The model under review builds one solid part; all positions refer to its coordinate system, in mm. Give positions to 0.01 mm unless a question says otherwise; leave off trailing zeros.
Autodesk Inventor part; units mm, degrees
ref_plane "YZ Plane" through (0, 0, 0) normal (1, 0, 0) x (0, 1, 0)
ref_plane "XZ Plane" through (0, 0, 0) normal (0, 1, 0) x (-1, 0, 0)
ref_plane "XY Plane" through (0, 0, 0) normal (0, 0, 1) x (1, 0, 0)
sketch "Sketch1" plane through (0, 0, 0) normal (0, 0, 1) x (1, 0, 0)
  line L0 (-412.8165, 301.8597) -> (87.1835, 301.8597)
  line L1 (-427.8165, 301.8597) -> (-412.8165, 301.8597)
  line L2 (-427.8165, 286.8597) -> (-427.8165, 301.8597)
  line L3 (-427.8165, -73.1403) -> (-427.8165, 286.8597)
  line L4 (-412.8165, 286.8597) -> (-427.8165, 286.8597)
  line L5 (-412.8165, 286.8597) -> (-427.8165, 286.8597)
  line L6 (-412.8165, 301.8597) -> (-412.8165, 286.8597)
  line L7 (-427.8165, 301.8597) -> (-412.8165, 301.8597)
  line L8 (-427.8165, 286.8597) -> (-427.8165, 301.8597)
  line L9 (-412.8165, -88.1403) -> (-412.8165, -73.1403)
  line L10 (-412.8165, -73.1403) -> (-427.8165, -73.1403)
  line L11 (-427.8165, -88.1403) -> (-427.8165, -73.1403)
  line L12 (-412.8165, -88.1403) -> (-427.8165, -88.1403)
  line L13 (-412.8165, -73.1403) -> (-412.8165, 286.8597)
  line L14 (87.1835, -73.1403) -> (-412.8165, -73.1403)
  line L15 (87.1835, -88.1403) -> (-412.8165, -88.1403)
  line L16 (102.1835, -88.1403) -> (102.1835, -73.1403)
  line L17 (102.1835, -73.1403) -> (87.1835, -73.1403)
  line L18 (87.1835, -88.1403) -> (87.1835, -73.1403)
  line L19 (102.1835, -88.1403) -> (87.1835, -88.1403)
  line L20 (87.1835, -73.1403) -> (87.1835, 286.8597)
  line L21 (102.1835, -73.1403) -> (102.1835, 286.8597)
  line L22 (87.1835, 286.8597) -> (102.1835, 286.8597)
  line L23 (102.1835, 286.8597) -> (102.1835, 301.8597)
  line L24 (87.1835, 301.8597) -> (102.1835, 301.8597)
  line L25 (87.1835, 286.8597) -> (87.1835, 301.8597)
  line L26 (87.1835, 286.8597) -> (-412.8165, 286.8597)
  line L27 (-312.8165, -73.1403) -> (-312.8165, 286.8597)
  line L28 (-297.8165, -73.1403) -> (-297.8165, 286.8597)
  line L29 (-12.8165, -73.1403) -> (-12.8165, 286.8597)
  line L30 (-27.8165, -73.1403) -> (-27.8165, 286.8597)
  line L31 (-425.8165, -71.1403) -> (-410.8165, -71.1403)
  line L32 (-410.8165, -71.1403) -> (-410.8165, -86.1403)
  line L33 (-410.8165, -86.1403) -> (85.1835, -86.1403)
  line L34 (85.1835, -86.1403) -> (85.1835, -71.1403)
  line L35 (85.1835, -71.1403) -> (100.1835, -71.1403)
  line L36 (100.1835, -71.1403) -> (100.1835, 284.8597)
  line L37 (100.1835, 284.8597) -> (85.1835, 284.8597)
  line L38 (85.1835, 284.8597) -> (85.1835, 299.8597)
  line L39 (85.1835, 299.8597) -> (-410.8165, 299.8597)
  line L40 (-410.8165, 299.8597) -> (-410.8165, 284.8597)
  line L41 (-410.8165, 284.8597) -> (-425.8165, 284.8597)
  line L42 (-425.8165, 284.8597) -> (-425.8165, -71.1403)
  point P0 (0, 0)
  dimension "d2" = 2
  dimension "d3" = 2
  dimension "d4" = 2
  dimension "d5" = 2
  dimension "d6" = 2
  dimension "d7" = 2
  dimension "d8" = 2
  dimension "d9" = 2
  dimension "d10" = 2
  dimension "d11" = 2
  dimension "d12" = 2
  dimension "d13" = 2
extrude "Extrusion1" add sketch "Sketch1" along normal blind 3 contours L41 L40 L26 L27 L14 L32 L31 L13 | L13 L31 L42 L41 | L40 L39 L38 L26 | L37 L36 L35 L20 | L20 L35 L34 L14 L29 L26 L38 L37 | L26 L28 L14 L27 | L29 L14 L30 L26 | L26 L30 L14 L28 | L14 L34 L33 L32
sketch "Sketch3" plane through (0, 0, 3) normal (0, 0, 1) x (1, 0, 0)
  line L0 (100.1835, -71.1403) -> (100.1835, 284.8597)
  line L1 (-425.8165, 284.8597) -> (-425.8165, -71.1403)
  line L2 (-425.8165, -71.1403) -> (-410.8165, -71.1403)
  line L3 (-410.8165, 284.8597) -> (-425.8165, 284.8597)
  line L4 (85.1835, -86.1403) -> (85.1835, -71.1403)
  line L5 (-410.8165, 299.8597) -> (-410.8165, 284.8597)
  line L6 (-410.8165, -86.1403) -> (85.1835, -86.1403)
  line L7 (85.1835, 299.8597) -> (-410.8165, 299.8597)
  point P0 (0, 0)
  point P1 (94.6835, -21.1403)
  point P2 (94.6835, 106.8597)
  point P3 (94.6835, 234.8597)
  point P4 (-420.3165, 234.8597)
  point P5 (-420.3165, 106.8597)
  point P6 (-420.3165, -21.1403)
  point P7 (35.1835, -80.6403)
  point P8 (-94.8165, -80.6403)
  point P9 (-230.8165, -80.6403)
  point P10 (-360.8165, -80.6403)
  point P11 (-360.8165, 294.3597)
  point P12 (-230.8165, 294.3597)
  point P13 (-94.8165, 294.3597)
  point P14 (35.1835, 294.3597)
  dimension "d18" = 5.5
  dimension "d19" = 5.5
  dimension "d20" = 50
  dimension "d21" = 50
  dimension "d22" = 356
  dimension "d23" = 178
  dimension "d24" = 50
  dimension "d25" = 50
  dimension "d26" = 5.5
  dimension "d27" = 5.5
  dimension "d28" = 180
  dimension "d29" = 180
hole "FrameMountHoles" at (94.6835, -21.1403, 3) at (94.6835, 106.8597, 3) at (94.6835, 234.8597, 3) at (-420.3165, 234.8597, 3) at (-420.3165, 106.8597, 3) at (-420.3165, -21.1403, 3) at (35.1835, -80.6403, 3) at (-94.8165, -80.6403, 3) at (-230.8165, -80.6403, 3) at (-360.8165, -80.6403, 3) at (-360.8165, 294.3597, 3) at (-230.8165, 294.3597, 3) at (-94.8165, 294.3597, 3) at (35.1835, 294.3597, 3) direction (0, 0, -1) diameter 4 depth 8 tip angle 118
sketch "Sketch10" plane through (0, 0, 3) normal (0, 0, 1) x (1, 0, 0)
  circle A0 centre (-94.8165, 294.3597) radius 2
  circle A1 centre (-360.8165, 294.3597) radius 2
  circle A2 centre (-230.8165, -80.6403) radius 2
  circle A3 centre (35.1835, -80.6403) radius 2
  circle A4 centre (-420.3165, 106.8597) radius 2
  circle A5 centre (94.6835, 234.8597) radius 2
  circle A6 centre (94.6835, -21.1403) radius 2
  circle A7 centre (94.6835, 106.8597) radius 2
  circle A8 centre (-420.3165, 234.8597) radius 2
  circle A9 centre (-420.3165, -21.1403) radius 2
  circle A10 centre (-94.8165, -80.6403) radius 2
  circle A11 centre (-360.8165, -80.6403) radius 2
  circle A12 centre (-230.8165, 294.3597) radius 2
  circle A13 centre (35.1835, 294.3597) radius 2
  line L0 (-425.8165, -71.1403) -> (-410.8165, -71.1403)
  line L1 (-410.8165, -71.1403) -> (-410.8165, -86.1403)
  line L2 (-410.8165, -86.1403) -> (85.1835, -86.1403)
  line L3 (85.1835, -86.1403) -> (85.1835, -71.1403)
  line L4 (85.1835, -71.1403) -> (100.1835, -71.1403)
  line L5 (100.1835, -71.1403) -> (100.1835, 284.8597)
  line L6 (100.1835, 284.8597) -> (85.1835, 284.8597)
  line L7 (85.1835, 284.8597) -> (85.1835, 299.8597)
  line L8 (85.1835, 299.8597) -> (-410.8165, 299.8597)
  line L9 (-410.8165, 299.8597) -> (-410.8165, 284.8597)
  line L10 (-410.8165, 284.8597) -> (-425.8165, 284.8597)
  line L11 (-425.8165, 284.8597) -> (-425.8165, -71.1403)
  line L12 (100.1835, -71.1403) -> (100.1835, 284.8597)
  line L13 (85.1835, 284.8597) -> (100.1835, 284.8597)
  line L14 (100.1835, 284.8597) -> (100.1835, 266.8597)
  line L15 (100.1835, 266.8597) -> (85.1835, 266.8597)
  line L16 (85.1835, 266.8597) -> (85.1835, 284.8597)
  line L17 (85.1835, 284.8597) -> (67.1835, 284.8597)
  line L18 (67.1835, 284.8597) -> (67.1835, 299.8597)
  line L19 (67.1835, 299.8597) -> (85.1835, 299.8597)
  line L20 (85.1835, 299.8597) -> (85.1835, 284.8597)
  line L21 (-410.8165, 284.8597) -> (-392.8165, 284.8597)
  line L22 (-392.8165, 284.8597) -> (-392.8165, 299.8597)
  line L23 (-392.8165, 299.8597) -> (-410.8165, 299.8597)
  line L24 (-410.8165, 299.8597) -> (-410.8165, 284.8597)
  line L25 (-410.8165, 284.8597) -> (-425.8165, 284.8597)
  line L26 (-425.8165, 284.8597) -> (-425.8165, 266.8597)
  line L27 (-425.8165, 266.8597) -> (-410.8165, 266.8597)
  line L28 (-410.8165, 266.8597) -> (-410.8165, 284.8597)
  line L29 (-410.8165, -71.1403) -> (-425.8165, -71.1403)
  line L30 (-425.8165, -71.1403) -> (-425.8165, -53.1403)
  line L31 (-425.8165, -53.1403) -> (-410.8165, -53.1403)
  line L32 (-410.8165, -53.1403) -> (-410.8165, -71.1403)
  line L33 (-410.8165, -71.1403) -> (-392.8165, -71.1403)
  line L34 (-392.8165, -71.1403) -> (-392.8165, -86.1403)
  line L35 (-392.8165, -86.1403) -> (-410.8165, -86.1403)
  line L36 (-410.8165, -86.1403) -> (-410.8165, -71.1403)
  line L37 (-410.8165, -86.1403) -> (85.1835, -86.1403)
  line L38 (85.1835, -71.1403) -> (67.1835, -71.1403)
  line L39 (67.1835, -71.1403) -> (67.1835, -86.1403)
  line L40 (67.1835, -86.1403) -> (85.1835, -86.1403)
  line L41 (85.1835, -86.1403) -> (85.1835, -71.1403)
  line L42 (85.1835, -71.1403) -> (100.1835, -71.1403)
  line L43 (100.1835, -71.1403) -> (100.1835, -53.1403)
  line L44 (100.1835, -53.1403) -> (85.1835, -53.1403)
  line L45 (85.1835, -53.1403) -> (85.1835, -71.1403)
  point P0 (0, 0)
  dimension "d78" = 18
extrude "TriCuts" cut sketch "Sketch10" against normal through all contours L11 L31 L32 L0 | L33 L34 L2 L1 | L11 L10 L28 L27 | L39 L38 L3 L2 | L9 L8 L22 L21 | L45 L44 L5 L4 | L8 L7 L17 L18 | L15 L16 L6 L5
equation "\"d4\" = d2"
equation "\"d5\" = d3"
equation "\"d6\" = d2"
equation "\"d7\" = d2"
equation "\"d8\" = d3"
equation "\"d9\" = d2"
equation "\"d10\" = d2"
equation "\"d11\" = d3"
equation "\"d12\" = d2"
equation "\"d13\" = d2"
properties part number "BasePlate" material "Aluminum 6061"
Item 1: Clearance check with flat-ended pins moving along their axes: pin 1 Ø1.5 at (y, z) = (-77.5, 1) entering from +X; pin 2 Ø1.5 at (y, z) = (-58, 2) entering from -X; pin 3 Ø3 at (x, y) = (35.18, -80.64) entering from +Z; pin 4 Ø1.5 at (x, z) = (-403.5, 1.5) entering from +Y. State where each tip first meets the part, or that it passes through.
Values found:
pin 1: stops at x = 67.18
pin 2: stops at x = -410.82
pin 3: passes through
pin 4: stops at y = 284.86
Item 2: Take a section at A-A (z = 2.4). Give the number of separate pieces and of enclosed holes in the cut face, and give its area (3 significant figures).
Values found:
separate pieces: 1
enclosed holes: 14
area: 200,000 mm2
Item 3: For line 1 (Y direction, x = -403, z = 1.1); line 2 (X direction, y = -54.5, z = 1.4), list the stretches that pass through material, from the lowest coordinate up.
Values found:
line 1: y = -71.14 to 284.86
line 2: x = -410.82 to 85.18
